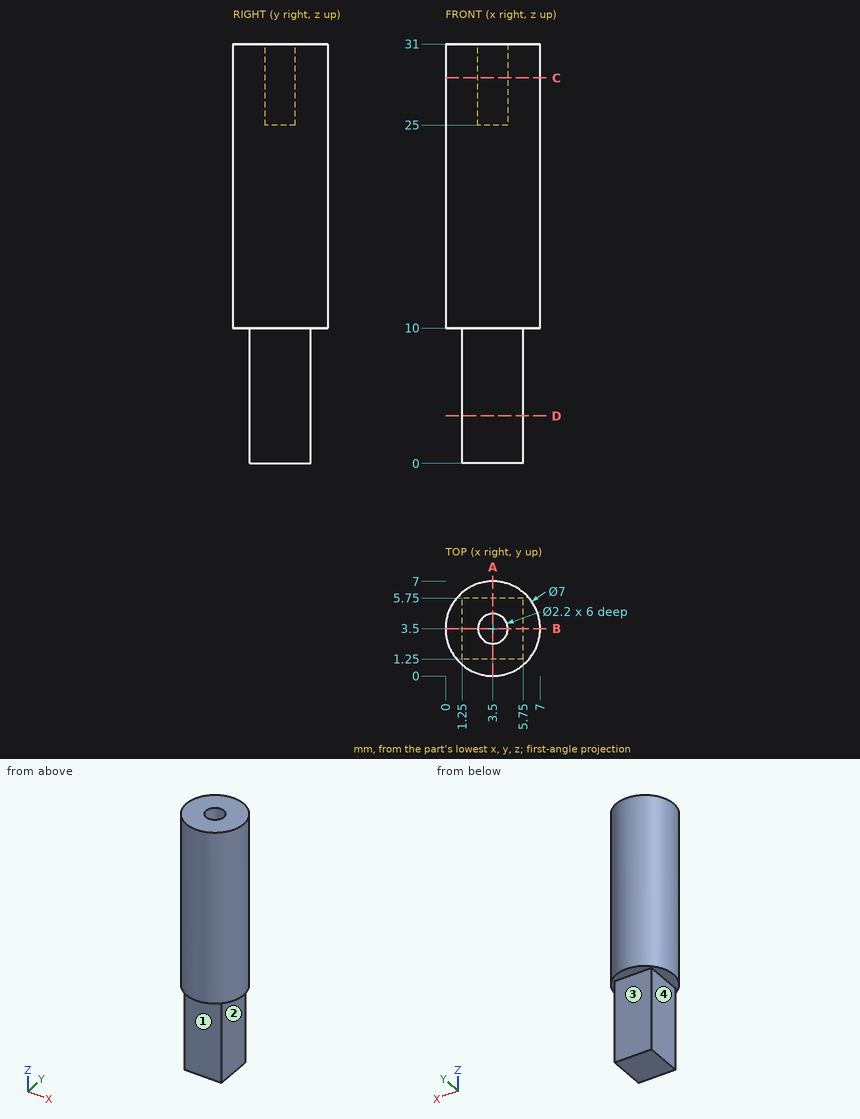
Verification items for this drawing (mm, ordinates from the low corner). A direction names the side the tool comes from. Coordinates: 2 decimals unless noted, no trailing zeros. Order: outer loops, then holes, each group sorted by start corner. A loop starts at its lowest first (then second) coordinate and runs counter-clockwise, first axis right, second up. Notation, with made-up numbers: M -13.75,1.25 L 41.25,1.25 A26 cw 41.25,37.25 Z; hole C 74,80.5 d5. An arc over 180 degrees is marked long. Answer as a JSON object with one key per item and string values.
Q1. Cross-section at D-D on z = 3.5. Record the cut outline in (x, y), and give its area (4 significant figures).
Results are:
{"outline": "M 1.25,1.25 L 5.75,1.25 L 5.75,5.75 L 1.25,5.75 Z", "area": "20.25 mm²"}
Q2. Scan lines: line 1 (Y direction, x = 3.5, z = 28.55); line 2 (Z direction, x = 6.25, y = 5.5); line 3 (Z direction, x = 3.5, y = 2.5). Record each from-to range of solid material in increasing order.
Results are:
{"line 1": "y = 0 to 2.4, 4.6 to 7", "line 2": "z = 10 to 31", "line 3": "z = 0 to 25"}
Q3. Cross-section at A-A on x = 3.5. Record the cut outline in (y, z).
Results are:
{"outline": "M 0,10 L 1.25,10 L 1.25,0 L 5.75,0 L 5.75,10 L 7,10 L 7,31 L 4.6,31 L 4.6,25 L 2.4,25 L 2.4,31 L 0,31 Z"}
Q4. Depth check by flat-ended pin: pin 1 Ø2 at (x, z) = (3.5, 6.5) entering from +Y; pin 2 Ø3.5 at (y, z) = (2.5, 7.5) entering from +X; pin 3 Ø2 at (y, z) = (5.5, 23) entering from +X. Enter the tip coordinate at first touch or a pass-through.
Results are:
{"pin 1": "stops at y = 5.75", "pin 2": "stops at x = 5.75", "pin 3": "stops at x = 6.85"}
Q5. Tool access check on the marked faces 1, 2, 3 and 4. Record the directions out of +Z, -Z, +X, -X, +Y, -Y that give a thin tool (end or side, any length) a straight path to the whole face; none if there is none.
Results are:
{"face 1": "-Z, +X, -X, -Y", "face 2": "-Z, +X, +Y, -Y", "face 3": "-Z, +X, -X, +Y", "face 4": "-Z, -X, +Y, -Y"}
Q6. Cross-section at C-C on z = 28.5. Record the cut outline in (x, y), and give its area (3 significant figures).
Results are:
{"outline": "C 3.5,3.5 d7; hole C 3.5,3.5 d2.2", "area": "34.7 mm²"}
